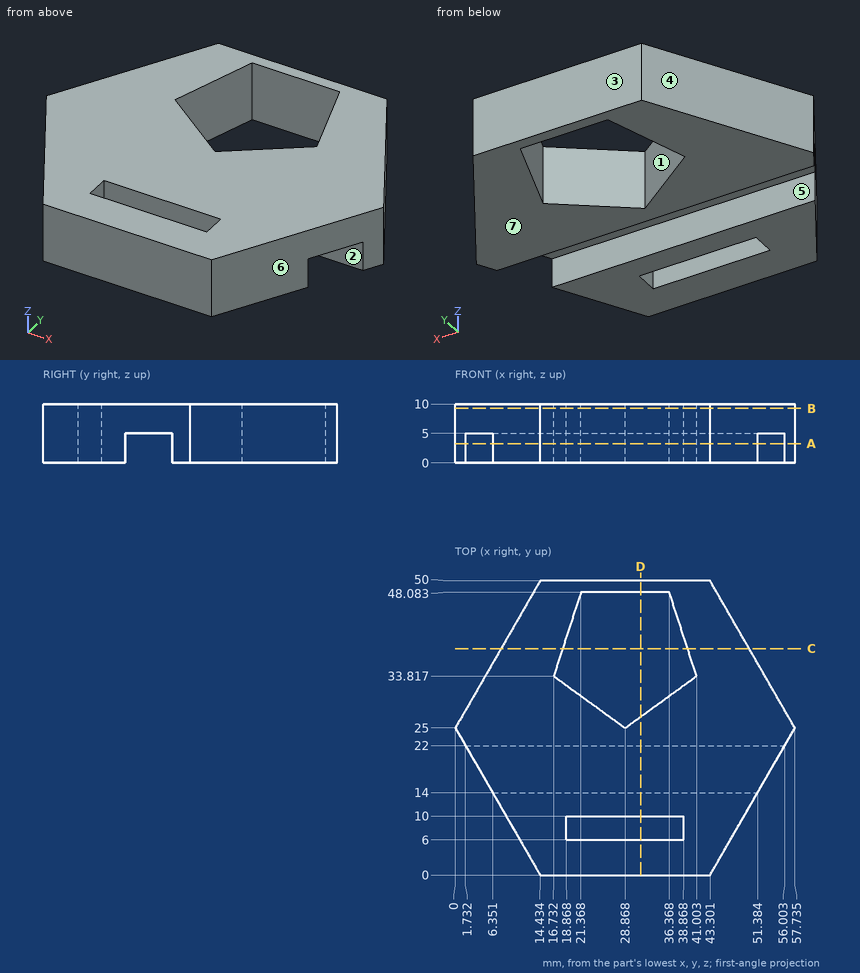
Geometry: see drawing. Coordinates: mm, zero at the bounding-box minimum. A direction names the side the tool comes from. Give positions to 0.01 mm unless a question says otherwise; leave off trailing zeros. Order: outer loops, then holes, each group sorted by start corner. A loop starts at its lowest first (then second) coordinate and runs counter-clockwise, first axis right, second up. Notation, with made-up numbers: (24, 71.5) - (74, 71.5) arc R28 cw to (74, 109.5) - close; hole circle Ø10 at (48, 39). An arc over 180 degrees is marked (long way). Use a Markdown table: item, result.
(1) Line query: line 1 (Y direction, x = 28.5, z = 7) (1 decimal); line 2 (Y direction, x = 26, z = 7.75) (1 decimal); line 3 (Y direction, x = 16, z = 3). Output: solid intervals per line, ascending. Write a range as from..to.
Computed values:
| item | result |
|---|---|
| line 1 | y = 0..6, 10..25.3, 48.1..50 |
| line 2 | y = 0..6, 10..27.1, 48.1..50 |
| line 3 | y = 0..14, 22..50 |
(2) Draft query along Y for the marked faces 4, 5, 6 and 7. Return one class per face: released by +Y, released by -Y, zero draft, split by the parting line, or undercut.
Computed values:
| item | result |
|---|---|
| face 4 | released by +Y |
| face 5 | undercut |
| face 6 | released by -Y |
| face 7 | zero draft |
(3) Section query A-A (z = 3.25). State how many separate pieces and enclosed holes the cut face has, then the cut area to 3 significant figures.
Computed values:
| item | result |
|---|---|
| separate pieces | 2 |
| enclosed holes | 2 |
| area | 1,300 mm2 |
(4) Section query B-B (z = 9.25). Output: boundary loops of the cut face in (x, y) (1 decimal), then the cut area to 3 significant figures.
Computed values:
| item | result |
|---|---|
| outline | (0, 25) - (14.4, 0) - (43.3, 0) - (57.7, 25) - (43.3, 50) - (14.4, 50) - close; hole (16.7, 33.8) - (28.9, 25) - (41, 33.8) - (36.4, 48.1) - (21.4, 48.1) - close; hole (18.9, 6) - (38.9, 6) - (38.9, 10) - (18.9, 10) - close |
| area | 1,700 mm2 |
(5) Access query for the marked faces 1, 2 and 3. Directions: +Z, -Z, +X, -X, +Y, -Y. A direction counts if a zero-diameter tool reaches every point of the face in a straight line with its end or side. Return the directions, or none.
Computed values:
| item | result |
|---|---|
| face 1 | +Z, -Z |
| face 2 | -Z, +X, -X |
| face 3 | +Z, -Z, +X, -X, +Y |
(6) Section query D-D (x = 31.5). Output: boundary loops of the cut face in (y, z).
Computed values:
| item | result |
|---|---|
| outline | (0, 0) - (6, 0) - (6, 10) - (0, 10) - close; (10, 0) - (14, 0) - (14, 5) - (22, 5) - (22, 0) - (26.91, 0) - (26.91, 10) - (10, 10) - close; (48.08, 0) - (50, 0) - (50, 10) - (48.08, 10) - close |
(7) Pin query (flat end, axial travel): pin 1 (2 mm diameter, centred on y = 8.5, z = 5, fed in from -X); pin 2 (4 mm diameter, centred on x = 11.5, y = 19, fed in from -Z); pin 3 (5 mm diameter, centred on x = 49, z = 1.5, fed in from +Y). Return the tip coordinate at first contact, or that it passes through.
Computed values:
| item | result |
|---|---|
| pin 1 | stops at x = 8.95 |
| pin 2 | stops at z = 5 |
| pin 3 | stops at y = 44.46 |
(8) Section query C-C (y = 38.5). Output: boundary loops of the cut face in (x, z) (1 decimal), then the cut area to 3 significant figures.
Computed values:
| item | result |
|---|---|
| outline | (7.8, 0) - (18.3, 0) - (18.3, 10) - (7.8, 10) - close; (39.5, 0) - (49.9, 0) - (49.9, 10) - (39.5, 10) - close |
| area | 209 mm2 |
